from build123d import *

# Parameters (mm, degrees)
CORTAR_EXTRUIR1_START = -1.8
CORTAR_EXTRUIR1_DEPTH = 3


with BuildPart() as part:
    # Croquis1 → Revolución1 (revolve)
    with BuildSketch(Plane.XY):
        with BuildLine():
            Line((0, 0), (0, 11.9))
            ThreePointArc((0, 11.9), (1.620417383, 11.535759883), (3.032129542, 10.660835807))
            ThreePointArc((3.032129542, 10.660835807), (3.082244216, 10.59308012), (3.1, 10.510696592))
            Line((3.1, 10.510696592), (3.1, 9.7))
            ThreePointArc((3.1, 9.7), (3.041421356, 9.558578644), (2.9, 9.5))
            Line((2.9, 9.5), (1.6, 9.5))
            Line((1.6, 9.5), (1.6, 1.6))
            Line((1.6, 1.6), (0, 0))
        make_face()
    revolve(axis=Axis((0, 0, 0), (0, 1, 0)))

    # Croquis2 → Cortar-Extruir1 (cut)
    with BuildSketch(Plane.XZ.offset(-9.5).offset(CORTAR_EXTRUIR1_START)):
        with BuildLine():
            Line((-0.4, 3.2), (-0.4, 0.9))
            ThreePointArc((-0.4, 0.9), (-0.546446609, 0.546446609), (-0.9, 0.4))
            Line((-0.9, 0.4), (-3.2, 0.4))
            Line((-3.2, 0.4), (-3.2, -0.4))
            Line((-3.2, -0.4), (-0.9, -0.4))
            ThreePointArc((-0.9, -0.4), (-0.546446609, -0.546446609), (-0.4, -0.9))
            Line((-0.4, -0.9), (-0.4, -3.2))
            Line((-0.4, -3.2), (0.4, -3.2))
            Line((0.4, -3.2), (0.4, -0.9))
            ThreePointArc((0.4, -0.9), (0.546446609, -0.546446609), (0.9, -0.4))
            Line((0.9, -0.4), (3.2, -0.4))
            Line((3.2, -0.4), (3.2, 0.4))
            Line((3.2, 0.4), (0.9, 0.4))
            ThreePointArc((0.9, 0.4), (0.546446609, 0.546446609), (0.4, 0.9))
            Line((0.4, 0.9), (0.4, 3.2))
            Line((0.4, 3.2), (-0.4, 3.2))
        make_face()
    extrude(amount=-CORTAR_EXTRUIR1_DEPTH, mode=Mode.SUBTRACT)


solid = part.part
Build history of the part. All positions in model axes, mm. Give positions to 0.01 mm unless a question says otherwise; leave off trailing zeros. Loops run counter-clockwise (first coordinate to the right, second up) from the corner with the lowest first, then second, coordinate; pieces in that order, holes last. Notation, with made-up numbers: (30.25, -0.5) -> (67.25, -0.5) arc R14 ccw to (67.25, 24.5) -> close; hole circle Ø11 at (85.25, 76). An arc over 180 degrees is marked (long way). Answer in a Markdown table with one row per item.
Item 1: Flat gauge pins, fed straight in: P1, Ø1, axis at x = 1.5, z = 2, coming from the +Y side; P2, Ø1.5, axis at x = -2, z = -1, coming from the +Y side; P3, Ø1.5, axis at x = 1, y = 7.5, coming from the +Z side. Where does each tip first touch, or does it go through?
Findings below:
| item | result |
|---|---|
| P1 | stops at y = 11.36 |
| P2 | stops at y = 11.59 |
| P3 | stops at z = 1.58 |
Item 2: Slice it at A-A on y = 4.25. Write the cut outline in (x, z), plus the area to 3 significant figures.
Findings below:
| item | result |
|---|---|
| outline | circle Ø3.2 at (0, 0) |
| area | 8.04 mm² |
Item 3: Slice it at B-B on y = 1. Write the cut outline in (x, z), plus the area to 3 significant figures.
Findings below:
| item | result |
|---|---|
| outline | circle Ø2 at (0, 0) |
| area | 3.14 mm² |
Item 4: Probe line 1 along Z through (x, y) = (0, 5.5); line 2 along Z through (x, y) = (1, 4.25); line 3 along X through (y, z) = (10.5, -0.5). List the from-to ranges inside material, lowest first. Write a range as [from, to].
Findings below:
| item | result |
|---|---|
| line 1 | z = [-1.6, 1.6] |
| line 2 | z = [-1.25, 1.25] |
| line 3 | x = [-3.06, 3.06] |
Item 5: Mould opens along X. For faces 1 (the flat face through (0, 11.3, 0)), 2 (the flat face through (1.25, 9.5, 1.25)), 3 (the cylindrical face through (1.43, 10.1, 2.75)) say: pulls with the +X half, pulls with the -X half, needs draft (parallel to the pull), parting line crosses it, or undercut.
Findings below:
| item | result |
|---|---|
| face 1 | undercut |
| face 2 | needs draft |
| face 3 | parting line crosses it |
